```python
from build123d import *

# Parameters (mm, degrees)
SKETCH1_W           = 150
SKETCH1_H           = 255
BASE_FLANGE1_DEPTH  = 4
CUT_EXTRUDE1_DEPTH  = 266.830773237
SKETCH5_W           = 4
SKETCH5_H           = 39
TAB1_DEPTH          = 4
SKETCH6_R           = 2.25
CUT_EXTRUDE2_DEPTH  = 267.986891064
TAB2_DEPTH          = 4
SKETCH8_R           = 1.75
CUT_EXTRUDE3_DEPTH  = 392.492017799
SKETCH10_R          = 1.75
SKETCH10_W          = 4.3
SKETCH10_H          = 20.5
CUT_EXTRUDE5_DEPTH  = 392.492017799
CUT_EXTRUDE6_DEPTH  = 392.492017799
SKETCH12_W          = 4.5
SKETCH12_H          = 21.5
CUT_EXTRUDE7_DEPTH  = 392.492017799
SKETCH14_R          = 1.75
CUT_EXTRUDE9_DEPTH  = 392.492017799
CUT_EXTRUDE11_DEPTH = 392.492017799
CUT_EXTRUDE12_DEPTH = 392.492017799


# Sheet-metal steps are written as plain solids
with BuildPart() as part:
    # Sketch1 → Base-Flange1 (new body)
    with BuildSketch(Plane(origin=(0, 0, 0), x_dir=(0, 0, -1), z_dir=(1, 0, 0))):
        with Locations((0, -127.5)):
            Rectangle(SKETCH1_W, SKETCH1_H)
    extrude(amount=-BASE_FLANGE1_DEPTH)

    # Sketch4 → Cut-Extrude1 (cut, through all)
    with BuildSketch(Plane(origin=(0, 0, 0), x_dir=(0, 0, -1), z_dir=(1, 0, 0))):
        Polygon((-75, -43.25), (-75, -46.75), (-72, -46.75), (-72, -47.75), (-68, -47.75), (-68, -46.75), (-63, -46.75), (-63, -43.25), (-68, -43.25), (-68, -42.25), (-72, -42.25), (-72, -43.25), align=None)
        Polygon((-72, -146.75), (-75, -146.75), (-75, -143.25), (-72, -143.25), (-72, -142.25), (-68, -142.25), (-68, -143.25), (-63, -143.25), (-63, -146.75), (-68, -146.75), (-68, -147.75), (-72, -147.75), align=None)
        Polygon((75, -146.75), (75, -143.25), (72, -143.25), (72, -142.25), (68, -142.25), (68, -143.25), (63, -143.25), (63, -146.75), (68, -146.75), (68, -147.75), (72, -147.75), (72, -146.75), align=None)
        Polygon((72, -43.25), (75, -43.25), (75, -46.75), (72, -46.75), (72, -47.75), (68, -47.75), (68, -46.75), (63, -46.75), (63, -43.25), (68, -43.25), (68, -42.25), (72, -42.25), align=None)
    extrude(amount=-CUT_EXTRUDE1_DEPTH, mode=Mode.SUBTRACT)

    # Sketch5 → Tab1 (add)
    with BuildSketch(Plane(origin=(0, 0, 0), x_dir=(0, 0, -1), z_dir=(1, 0, 0))):
        with Locations((-77, -95)):
            Rectangle(SKETCH5_W, SKETCH5_H)
        with Locations((77, -95)):
            Rectangle(SKETCH5_W, SKETCH5_H)
    extrude(amount=-TAB1_DEPTH)

    # Sketch6 → Cut-Extrude2 (cut, through all)
    with BuildSketch(Plane(origin=(0, 0, 0), x_dir=(0, 0, -1), z_dir=(1, 0, 0))):
        with Locations((-55, -14.5)):
            Circle(SKETCH6_R)
        with Locations(Location((55, -14.5, 0), (0, 0, 180))):
            Circle(SKETCH6_R)
    extrude(amount=-CUT_EXTRUDE2_DEPTH, mode=Mode.SUBTRACT)

    # Sketch7 → Tab2 (add)
    with BuildSketch(Plane(origin=(0, 0, 0), x_dir=(0, 0, -1), z_dir=(1, 0, 0))):
        Polygon((-75, -255), (-90, -270), (-90, -355), (-165, -355), (-165, -241.5), (-79, -155.5), (-75, -155.5), align=None)
        Polygon((75, -155.5), (75, -255), (90, -270), (90, -355), (165, -355), (165, -241.5), (79, -155.5), align=None)
    extrude(amount=-TAB2_DEPTH)

    # Sketch8 → Cut-Extrude3 (cut, through all)
    with BuildSketch(Plane(origin=(0, 0, 0), x_dir=(0, 0, -1), z_dir=(1, 0, 0))):
        with Locations((-77, -205)):
            Circle(SKETCH8_R)
        with Locations((77, -205)):
            Circle(SKETCH8_R)
    extrude(amount=-CUT_EXTRUDE3_DEPTH, mode=Mode.SUBTRACT)

    # Sketch10 → Cut-Extrude5 (cut, through all)
    with BuildSketch(Plane(origin=(0, 0, 0), x_dir=(0, 0, -1), z_dir=(1, 0, 0))):
        with Locations((-100, -299.75)):
            Circle(SKETCH10_R)
        with Locations((100, -299.75)):
            Circle(SKETCH10_R)
        with Locations((-100, -324.75)):
            Rectangle(SKETCH10_W, SKETCH10_H)
        with Locations((-100, -274.75)):
            Rectangle(SKETCH10_W, SKETCH10_H)
        with Locations((100, -274.75)):
            Rectangle(SKETCH10_W, SKETCH10_H)
        with Locations((100, -324.75)):
            Rectangle(SKETCH10_W, SKETCH10_H)
    extrude(amount=-CUT_EXTRUDE5_DEPTH, mode=Mode.SUBTRACT)

    # Sketch11 → Cut-Extrude6 (cut, through all)
    with BuildSketch(Plane(origin=(0, 0, 0), x_dir=(0, 0, -1), z_dir=(1, 0, 0))):
        Polygon((-20, 0), (-20, -4), (-1.75, -4), (-1.75, -7), (-2.75, -7), (-2.75, -11), (-1.75, -11), (-1.75, -16), (1.75, -16), (1.75, -11), (2.75, -11), (2.75, -7), (1.75, -7), (1.75, -4), (20, -4), (20, 0), align=None)
    extrude(amount=-CUT_EXTRUDE6_DEPTH, mode=Mode.SUBTRACT)

    # Sketch12 → Cut-Extrude7 (cut, through all)
    with BuildSketch(Plane(origin=(0, 0, 0), x_dir=(0, 0, -1), z_dir=(1, 0, 0))):
        with Locations((-77, -184.25)):
            Rectangle(SKETCH12_W, SKETCH12_H)
        with Locations((77, -184.25)):
            Rectangle(SKETCH12_W, SKETCH12_H)
    extrude(amount=-CUT_EXTRUDE7_DEPTH, mode=Mode.SUBTRACT)

    # Sketch14 → Cut-Extrude9 (cut, through all)
    with BuildSketch(Plane(origin=(-4, 0, 0), x_dir=(0, 1, 0), z_dir=(-1, 0, 0))):
        with Locations(Location((-172.7, 52.45, 0), (0, 0, 270))):
            Circle(SKETCH14_R)
        with Locations(Location((-172.7, -52.25, 0), (0, 0, 270))):
            Circle(SKETCH14_R)
        with Locations(Location((-86.7, -52.55, 0), (0, 0, 270))):
            Circle(SKETCH14_R)
        with Locations(Location((-87.2, 51.75, 0), (0, 0, 270))):
            Circle(SKETCH14_R)
    extrude(amount=-CUT_EXTRUDE9_DEPTH, mode=Mode.SUBTRACT)

    # Sketch16 → Cut-Extrude11 (cut, through all)
    with BuildSketch(Plane(origin=(0, 0, 0), x_dir=(0, 0, -1), z_dir=(1, 0, 0))):
        with BuildLine():
            Line((-74.75, -177.5), (-74.75, -191.5))
            ThreePointArc((-74.75, -191.5), (-70.693771456, -185.047817237), (-63.121014964, -185.906310995))
            ThreePointArc((-63.121014964, -185.906310995), (-55.125270956, -180.887787453), (-64.506473724, -179.833968012))
            ThreePointArc((-64.506473724, -179.833968012), (-70.559234361, -182.753028585), (-74.75, -177.5))
        make_face()
        with BuildLine():
            Line((74.75, -177.5), (74.75, -191.5))
            ThreePointArc((74.75, -191.5), (70.693771456, -185.047817237), (63.121014964, -185.906310995))
            ThreePointArc((63.121014964, -185.906310995), (55.125270956, -180.887787453), (64.506473724, -179.833968012))
            ThreePointArc((64.506473724, -179.833968012), (70.559234361, -182.753028585), (74.75, -177.5))
        make_face()
    extrude(amount=-CUT_EXTRUDE11_DEPTH, mode=Mode.SUBTRACT)

    # Sketch17 → Cut-Extrude12 (cut, through all)
    with BuildSketch(Plane(origin=(0, 0, 0), x_dir=(0, 0, -1), z_dir=(1, 0, 0))):
        with BuildLine():
            Line((52.45, -170.95), (52.95, -170.95))
            ThreePointArc((52.95, -170.95), (54.7, -172.7), (52.95, -174.45))
            Line((52.95, -174.45), (52.45, -174.45))
            ThreePointArc((52.45, -174.45), (50.7, -172.7), (52.45, -170.95))
        make_face()
        with BuildLine():
            Line((-51.532833161, -85.275966425), (-50.832833161, -85.775966425))
            ThreePointArc((-50.832833161, -85.775966425), (-50.425966425, -88.217166839), (-52.867166839, -88.624033575))
            Line((-52.867166839, -88.624033575), (-53.567166839, -88.124033575))
            ThreePointArc((-53.567166839, -88.124033575), (-53.974033575, -85.682833161), (-51.532833161, -85.275966425))
        make_face()
        with BuildLine():
            Line((50.967376208, -85.634752416), (51.967376208, -85.134752416))
            ThreePointArc((51.967376208, -85.134752416), (54.315247584, -85.917376208), (53.532623792, -88.265247584))
            Line((53.532623792, -88.265247584), (52.532623792, -88.765247584))
            ThreePointArc((52.532623792, -88.765247584), (50.184752416, -87.982623792), (50.967376208, -85.634752416))
        make_face()
    extrude(amount=-CUT_EXTRUDE12_DEPTH, mode=Mode.SUBTRACT)


solid = part.part
```
Can you work these out from the model? Positions are in its coordinate system, mm. A direction names the side the tool comes from. Give positions to 0.01 mm unless a question says otherwise; leave off trailing zeros. Write each loop counter-clockwise with the first axis right and the second up, starting at its lowest first coordinate (ties: lowest second). Pieces come first, ordered by that corner, then holes. Notation, with made-up numbers: (-19.5, 86.5) -> (15.5, 86.5) arc R6 ccw to (15.5, 93.5) -> close; hole circle Ø1 at (-37, 55). An arc over 180 degrees is marked (long way). One line per item, written item: value.
Q1. Imagine slicing it at A-A on y = -319. Please give me the cut outline in (x, z).
Results found:
outline: (-4, -165) -> (0, -165) -> (0, -102.15) -> (-4, -102.15) -> close; (-4, -97.85) -> (0, -97.85) -> (0, -90) -> (-4, -90) -> close; (-4, 90) -> (0, 90) -> (0, 97.85) -> (-4, 97.85) -> close; (-4, 102.15) -> (0, 102.15) -> (0, 165) -> (-4, 165) -> close
Q2. Which directions (+Z, -Z, +X, -X, +Y, -Y) give clear straight access to the entire face, cutting with the end or side of a thin tool? Please do faces 1 (the face through (-1.97, -181.06, 55.09)), 2 (the face through (-2, -262, 82)).
Results found:
face 1: +X, -X
face 2: +X, -X, -Y
Q3. Imagine slicing it at D-D on x = -0.65. Give the number of separate pieces and of enclosed holes in the cut face, and give its area (3 significant figures).
Results found:
separate pieces: 1
enclosed holes: 16
area: 63,000 mm^2
Q4. For P1, Ø2, axis at x = -3.5, z = -115, coming from the +Y side; P2, Ø2, axis at x = -2, z = 76, coming from the -Y side; P3, Ø0.5, axis at x = -1.5, y = -147.5, coming from the +Z side, each with a flat end and sliding along its axis, tell me the tip position at first contact or that it passes through.
Results found:
P1: stops at y = -190.5
P2: stops at y = -257
P3: stops at z = 75
Q5. Please list where these lines run through material, in increasing order: line 1 (Y direction, x = -2.3, z = 52.25); line 2 (Z direction, x = -1.1, y = -328.5); line 3 (Y direction, x = -2.15, z = -60). Write a range as [from, to].
Results found:
line 1: y = [-255, -174.45], [-170.95, -88.9], [-84.98, 0]
line 2: z = [-165, -102.15], [-97.85, -90], [90, 97.85], [102.15, 165]
line 3: y = [-255, -187], [-177, 0]
Q6. We'd pull the mould along Z, two halves only. Please class faces 3 (the face through (-1.97, -181.06, -55.09)), 4 (the face through (-2, -262, -82)), 5 (the face through (-2, -199.1, -122.6)), 6 (the face through (0, -175, -2)): +Z half, -Z half, draft (parallel to the pull), parting line (faces both ways), or undercut.
Results found:
face 3: undercut
face 4: undercut
face 5: -Z half
face 6: draft
Q7. Imagine slicing it at C-C on y = -56.5. Please give me the cut outline in (x, z).
Results found:
outline: (-4, -75) -> (0, -75) -> (0, 75) -> (-4, 75) -> close
Q8. Imagine slicing it at B-B on z = -33. Please give me the cut outline in (x, y).
Results found:
outline: (-4, -255) -> (0, -255) -> (0, 0) -> (-4, 0) -> close
